```python
from build123d import *

# Parameters (mm, degrees)
F0_R     = 31.75
F0_R_2   = 11.1125
F1_DEPTH = 12.7
F3_DEPTH = 25.4
F4_R     = 3.175
F5_DEPTH = 25.4


with BuildPart() as f1:
    # F0 (on Top) → F1 (new body)
    with BuildSketch(Plane.XY):
        Circle(F0_R)
        Circle(F0_R_2, mode=Mode.SUBTRACT)
    extrude(amount=F1_DEPTH)

    # F2 (on Top) → F3 (cut)
    with BuildSketch(Plane.XY):
        with BuildLine():
            ThreePointArc((8.7188916363, -37.0889596596), (19.05, -32.9955678842), (27.760535447, -26.0952614797))
            ThreePointArc((27.760535447, -26.0952614797), (13.49375, -23.3718605846), (8.7188916363, -37.0889596596))
        make_face()
        with BuildLine():
            ThreePointArc((-27.760535447, -26.0952614797), (-19.05, -32.9955678842), (-8.7188916363, -37.0889596596))
            ThreePointArc((-8.7188916363, -37.0889596596), (-8.1345957944, -35.0792202734), (-7.9375, -32.9955678842))
            ThreePointArc((-7.9375, -32.9955678842), (-15.396793799, -22.500724355), (-27.760535447, -26.0952614797))
        make_face()
        with BuildLine():
            ThreePointArc((-26.9875, 0), (-29.68880886, 7.2621980045), (-36.4794270833, 10.9936981799))
            ThreePointArc((-36.4794270833, 10.9936981799), (-38.1, 0), (-36.4794270833, -10.9936981799))
            ThreePointArc((-36.4794270833, -10.9936981799), (-29.68880886, -7.2621980045), (-26.9875, 0))
        make_face()
        with BuildLine():
            ThreePointArc((-7.9375, 32.9955678842), (-8.1345957944, 35.0792202734), (-8.7188916363, 37.0889596596))
            ThreePointArc((-8.7188916363, 37.0889596596), (-19.05, 32.9955678842), (-27.760535447, 26.0952614797))
            ThreePointArc((-27.760535447, 26.0952614797), (-15.396793799, 22.500724355), (-7.9375, 32.9955678842))
        make_face()
        with BuildLine():
            ThreePointArc((8.7188916363, 37.0889596596), (13.49375, 23.3718605846), (27.760535447, 26.0952614797))
            ThreePointArc((27.760535447, 26.0952614797), (19.05, 32.9955678842), (8.7188916363, 37.0889596596))
        make_face()
        with BuildLine():
            ThreePointArc((36.4794270833, -10.9936981799), (37.6926794741, -5.55625), (38.1, 0))
            ThreePointArc((38.1, 0), (37.6926794741, 5.55625), (36.4794270833, 10.9936981799))
            ThreePointArc((36.4794270833, 10.9936981799), (26.9875, 0), (36.4794270833, -10.9936981799))
        make_face()
    extrude(amount=F3_DEPTH, mode=Mode.SUBTRACT)

    # F4 (on Top) → F5 (cut)
    with BuildSketch(Plane.XY):
        with Locations((0, 22.86)):
            Circle(F4_R)
        with Locations((-19.7973407305, 11.43)):
            Circle(F4_R)
        with Locations((-19.7973407305, -11.43)):
            Circle(F4_R)
        with Locations((0, -22.86)):
            Circle(F4_R)
        with Locations((19.7973407305, -11.43)):
            Circle(F4_R)
        with Locations((19.7973407305, 11.43)):
            Circle(F4_R)
    extrude(amount=F5_DEPTH, mode=Mode.SUBTRACT)


solid = f1.part
```
For this review, take the finished solid that the model builds, in its own axes (mm). Coordinates: 2 decimals unless noted, no trailing zeros. Loops run counter-clockwise (first coordinate to the right, second up) from the corner with the lowest first, then second, coordinate; pieces in that order, holes last.
1. Add section A-A, the plane x = 0. Count the separate pieces of the cut face and the enclosed holes in it, then the cut area to 3 significant figures.
2. For line 1 (Y direction, x = 22.5, z = 8.5); line 2 (X direction, y = 11.43, z = 4); line 3 (Y direction, x = 1, z = 11.75), list the stretches that pass through material, from the lowest coordinate up.
3. Add section D-D, the plane x = -21. Give the boundary of the cut face in (y, z).
4. Mouldability with a two-part tool opening along Y and no side actions: class faces 1 (the cylindrical face through (27.554, 15.775, 6.261)), 2 (the cylindrical face through (22.826, -10.476, 6.261)), 3 (the cylindrical face through (27.438, -15.975, 6.261)) as +Y half, -Y half, draft (parallel to the pull), parting line (faces both ways), or undercut.
5. Insertion check: P1, Ø3, axis at x = -5.5, z = 1.5, coming from the -Y side; P2, Ø1.5, axis at y = -2.5, z = 7.5, coming from the +X side; P3, Ø3, axis at y = 5.5, z = 4, coming from the +X side. Each pin has a flat end and moves straight along its axis. Give the tip position at first contact, or say it passes through.
6. Add section C-C, the plane y = -6. Give the boundary of the cut face in (x, z), then the cut area to 3 significant figures.
Result:
1. separate pieces: 4
1. enclosed holes: 0
1. area: 363 mm2
2. line 1: y = -22.4 to -13.1, -9.76 to 9.76, 13.1 to 22.4
2. line 2: x = -29.62 to -22.97, -16.62 to 16.62, 22.97 to 29.62
2. line 3: y = -31.73 to -25.87, -19.85 to -11.07, 11.07 to 19.85, 25.87 to 31.73
3. outline: (-22.06, 0) - (-14.37, 0) - (-14.37, 12.7) - (-22.06, 12.7) - close; (-8.49, 0) - (8.49, 0) - (8.49, 12.7) - (-8.49, 12.7) - close; (14.37, 0) - (22.06, 0) - (22.06, 12.7) - (14.37, 12.7) - close
4. face 1: +Y half
4. face 2: undercut
4. face 3: -Y half
5. P1: stops at y = -31.5
5. P2: stops at x = 27.47
5. P3: stops at x = 29.47
6. outline: (-28.75, 0) - (-9.35, 0) - (-9.35, 12.7) - (-28.75, 12.7) - close; (9.35, 0) - (28.75, 0) - (28.75, 12.7) - (9.35, 12.7) - close
6. area: 493 mm2
